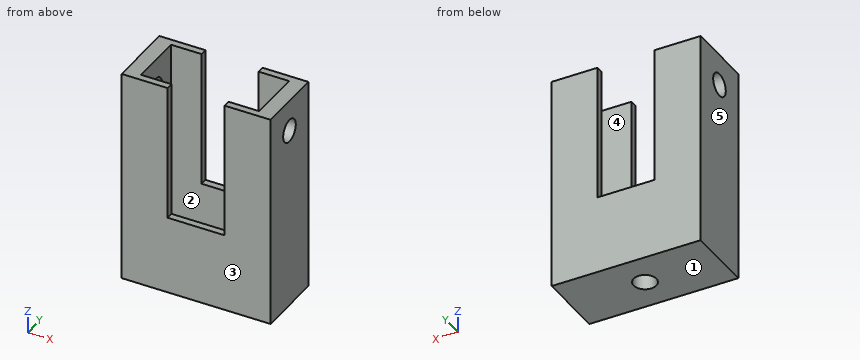
```python
from build123d import *

# Parameters (mm, degrees)
SKETCH2_W           = 65.5
SKETCH2_H           = 30
SKETCH2_W_2         = 52
SKETCH2_H_2         = 23.816793894
BOSS_EXTRUDE1_DEPTH = 94.5
SKETCH3_W           = 52
SKETCH3_H           = 23.816793894
BOSS_EXTRUDE2_DEPTH = 10
SKETCH4_W           = 25
SKETCH4_H           = 30
CUT_EXTRUDE1_DEPTH  = 60
SKETCH5_R           = 5
CUT_EXTRUDE2_DEPTH  = 116.954732547
SKETCH6_R           = 5
CUT_EXTRUDE3_DEPTH  = 102.132648042


with BuildPart() as part:
    # Sketch2 → Boss-Extrude1 (new body)
    with BuildSketch(Plane.XY):
        Rectangle(SKETCH2_W, SKETCH2_H)
        Rectangle(SKETCH2_W_2, SKETCH2_H_2, mode=Mode.SUBTRACT)
    extrude(amount=BOSS_EXTRUDE1_DEPTH)

    # Sketch3 → Boss-Extrude2 (add)
    with BuildSketch(Plane(origin=(0, 0, 0), x_dir=(-1, 0, 0), z_dir=(0, 0, -1))):
        Rectangle(SKETCH3_W, SKETCH3_H)
    extrude(amount=-BOSS_EXTRUDE2_DEPTH)

    # Sketch4 → Cut-Extrude1 (cut)
    with BuildSketch(Plane.XY.offset(94.5)):
        Rectangle(SKETCH4_W, SKETCH4_H)
    extrude(amount=-CUT_EXTRUDE1_DEPTH, mode=Mode.SUBTRACT)

    # Sketch5 → Cut-Extrude2 (cut, through all)
    with BuildSketch(Plane.ZY.offset(32.75)):
        with Locations(Location((80.690823626, 0, 0), (0, 0, 270))):
            Circle(SKETCH5_R)
    extrude(amount=-CUT_EXTRUDE2_DEPTH, mode=Mode.SUBTRACT)

    # Sketch6 → Cut-Extrude3 (cut, through all)
    with BuildSketch(Plane(origin=(0, 0, 0), x_dir=(-1, 0, 0), z_dir=(0, 0, -1))):
        Circle(SKETCH6_R)
    extrude(amount=-CUT_EXTRUDE3_DEPTH, mode=Mode.SUBTRACT)


solid = part.part
```
Geometry check sheet. Reference: the model listing, model coordinates, mm. Face numbers are marked on the shaded views. A direction names the side the tool comes from. Coordinates: 2 decimals unless noted, no trailing zeros. Write each loop counter-clockwise with the first axis right and the second up, starting at its lowest first coordinate (ties: lowest second). Pieces come first, ordered by that corner, then holes. Notation, with made-up numbers: M 52,30.5 L 96,30.5 A27 ccw 96,46.5 Z; hole C -19.75,87.25 d3. An arc over 180 degrees is marked long. Use one line per item in the form item = value. Start each with the question number.
1) Thickness scan on probe 1 along X at (y, z) = (-11.25, 73.5); probe 2 along Z at (x, y) = (28.5, 0); probe 3 along X at (y, z) = (-12.75, 73). Record the ranges inside material, lowest first. Write a range as from..to.
2) Section check D-D on x = -19.5. Enter the section's corners in (y, z).
3) Go/stop test with flat-tipped pins: pin 1 Ø0.9 at (x, y) = (-6, 13.5) entering from +Z; pin 2 Ø5 at (x, y) = (10.5, 7) entering from -Z; pin 3 Ø3 at (x, y) = (17.5, -0.5) entering from +Z. Record where each tip stops, or that it passes through.
4) Section check B-B on y = 0. Enter the section's corners in (x, z), and give its area (3 significant figures).
5) Section check C-C on x = 0. Enter the section's corners in (y, z).
6) Release check for a two-part mould opening along X. For the marked faces 3, 4 and 5 record: pulls with the +X half, pulls with the -X half, needs draft (parallel to the pull), parting line crosses it, or undercut.
7) Set-up check for the marked faces 1 and 2: record each of +Z, -Z, +X, -X, +Y, -Y from which the full face is reachable in a straight line by a thin tool's end or side.
8) Section check A-A on z = 46.5. Enter the section's corners in (x, y).
Responses:
q1.probe_1 = -32.75..-26, 26..32.75
q1.probe_2 = 0..75.69, 85.69..94.5
q1.probe_3 = -32.75..-12.5, 12.5..32.75
q2.outline = M -15,0 L 15,0 L 15,94.5 L 11.91,94.5 L 11.91,10 L -11.91,10 L -11.91,94.5 L -15,94.5 Z
q3.pin_1 = 34.5
q3.pin_2 = 0
q3.pin_3 = 10
q4.outline = M -32.75,0 L -5,0 L -5,10 L -26,10 L -26,75.69 L -32.75,75.69 Z; M -32.75,85.69 L -26,85.69 L -26,94.5 L -32.75,94.5 Z; M 5,0 L 32.75,0 L 32.75,75.69 L 26,75.69 L 26,10 L 5,10 Z; M 26,85.69 L 32.75,85.69 L 32.75,94.5 L 26,94.5 Z
q4.area = 1,560 mm2
q5.outline = M -15,0 L -5,0 L -5,10 L -11.91,10 L -11.91,34.5 L -15,34.5 Z; M 5,0 L 15,0 L 15,34.5 L 11.91,34.5 L 11.91,10 L 5,10 Z
q6.face_3 = needs draft
q6.face_4 = undercut
q6.face_5 = pulls with the -X half
q7.face_1 = -Z, +X, -X, +Y, -Y
q7.face_2 = +Z
q8.outline = M -32.75,-15 L -12.5,-15 L -12.5,-11.91 L -26,-11.91 L -26,11.91 L -12.5,11.91 L -12.5,15 L -32.75,15 Z; M 12.5,-15 L 32.75,-15 L 32.75,15 L 12.5,15 L 12.5,11.91 L 26,11.91 L 26,-11.91 L 12.5,-11.91 Z
